Part model, mm, in its own coordinate system. Face numbers are marked on the shaded views. A direction names the side the tool comes from. Round coordinates to 2 decimals unless told otherwise and drop trailing zeros. Loops run counter-clockwise (first coordinate to the right, second up) from the corner with the lowest first, then second, coordinate; pieces in that order, holes last. Notation, with made-up numbers: (83.25, 18.5) - (135.25, 18.5) arc R5 cw to (135.25, 27.5) - close; hole circle Ø5 at (0.5, 62.5). An arc over 180 degrees is marked (long way). Put each result on its own line as item: value.
Autodesk Inventor part; units mm, degrees
ref_plane "YZ Plane" through (0, 0, 0) normal (1, 0, 0) x (0, 1, 0)
ref_plane "XZ Plane" through (0, 0, 0) normal (0, 1, 0) x (-1, 0, 0)
ref_plane "XY Plane" through (0, 0, 0) normal (0, 0, 1) x (1, 0, 0)
sketch "スケッチ1" plane through (0, 0, 0) normal (1, 0, 0) x (0, 1, 0)
  circle A0 centre (0, 0) radius 5
  circle A1 centre (0, 0) radius 9.5
  dimension "d0" = 10
  dimension "d1" = 19
extrude "押し出し1" add sketch "スケッチ1" along normal blind 7
sketch "スケッチ2" plane through (7, 0, 0) normal (1, 0, 0) x (0, 0, -1)
  circle A0 centre (0, 0) radius 6
  circle A1 centre (0, 0) radius 7.5
  dimension "d4" = 12
  dimension "d5" = 15
extrude "押し出し2" cut sketch "スケッチ2" against normal blind 0.5
sketch "スケッチ3" plane through (0, 0, 0) normal (-1, 0, 0) x (0, 0, 1)
  circle A0 centre (0, 0) radius 6
  circle A1 centre (0, 0) radius 7.5
  dimension "d8" = 12
  dimension "d9" = 15
extrude "押し出し3" cut sketch "スケッチ3" against normal blind 0.5
properties part number "Bearing_626ZZ" material "ステンレス鋼"
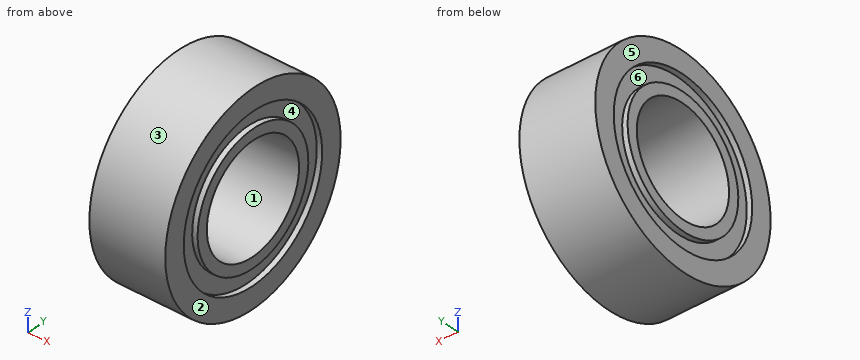
1. Band-saw the part on A-A (y = 0). List the corners of the cut face in (x, z), plus the area to 3 significant figures.
A:
outline: (0, -9.5) - (7, -9.5) - (7, -7.5) - (6.5, -7.5) - (6.5, -6) - (7, -6) - (7, -5) - (0, -5) - (0, -6) - (0.5, -6) - (0.5, -7.5) - (0, -7.5) - close; (0, 5) - (7, 5) - (7, 6) - (6.5, 6) - (6.5, 7.5) - (7, 7.5) - (7, 9.5) - (0, 9.5) - (0, 7.5) - (0.5, 7.5) - (0.5, 6) - (0, 6) - close
area: 60.0 mm²
2. Band-saw the part on C-C (x = 6.75). List the corners of the cut face in (y, z).
A:
outline: circle Ø19 at (0, 0); circle Ø12 at (0, 0); hole circle Ø15 at (0, 0); hole circle Ø10 at (0, 0)
3. Probe line 1 along Z through (x, y) = (4, 0); line 2 along Z through (x, y) = (1.75, -1.25); line 3 along Y through (x, z) = (1.5, -3.5). List the from-to ranges inside material, lowest first. Write a range as [from, to].
A:
line 1: z = [-9.5, -5], [5, 9.5]
line 2: z = [-9.42, -4.84], [4.84, 9.42]
line 3: y = [-8.83, -3.57], [3.57, 8.83]
4. Band-saw the part on D-D (x = 2.5). List the corners of the cut face in (y, z), plus the area to 3 significant figures.
A:
outline: circle Ø19 at (0, 0); hole circle Ø10 at (0, 0)
area: 205 mm²
5. Two-plate mould, pull along Y, no slides. Class the marked faces 1, 2, 3 and 4: pulls with the +Y half, pulls with the -Y half, needs draft (parallel to the pull), parting line crosses it, or undercut.
A:
face 1: undercut
face 2: needs draft
face 3: parting line crosses it
face 4: undercut
6. Pin check, flat tips, straight feed: P1, Ø9, axis at y = 0, z = 0, coming from the -X side; P2, Ø3, axis at x = 3.5, z = 4, coming from the +Y side; P3, Ø1, axis at x = 3.5, y = -4, coming from the -Z side; P4, Ø4.5, axis at y = -1, z = 3, coming from the -X side. Stop position of each tip, or through.
A:
P1: passes through
P2: stops at y = 9.17
P3: stops at z = -8.83
P4: stops at x = 0
7. Tool access for the marked faces 5 and 6: list every direction of +Z, -Z, +X, -X, +Y, -Y with a clear straight run to the whole face (end or side of a thin tool).
A:
face 5: +Z, -Z, -X, +Y, -Y
face 6: -X
